Autodesk Inventor part; units mm, degrees
ref_plane "YZ Plane" through (0, 0, 0) normal (1, 0, 0) x (0, 1, 0)
ref_plane "XZ Plane" through (0, 0, 0) normal (0, 1, 0) x (-1, 0, 0)
ref_plane "XY Plane" through (0, 0, 0) normal (0, 0, 1) x (1, 0, 0)
sketch "Sketch1" plane through (0, 0, 0) normal (0, 0, 1) x (1, 0, 0)
  line L0 (-21.15, 15.4985) -> (-15.4985, 21.15)
  line L1 (-15.4985, 21.15) -> (15.4985, 21.15)
  line L2 (15.4985, 21.15) -> (21.15, 15.4985)
  line L3 (21.15, 15.4985) -> (21.15, -15.4985)
  line L4 (21.15, -15.4985) -> (15.4985, -21.15)
  line L5 (15.4985, -21.15) -> (-15.4985, -21.15)
  line L6 (-15.4985, -21.15) -> (-21.15, -15.4985)
  line L7 (-21.15, -15.4985) -> (-21.15, 15.4985)
  line L8 (28.575, -18.574) -> (28.575, 18.574)
  line L9 (28.575, 18.574) -> (18.574, 28.575)
  line L10 (18.574, 28.575) -> (-18.574, 28.575)
  line L11 (-18.574, 28.575) -> (-28.575, 18.574)
  line L12 (-28.575, 18.574) -> (-28.575, -18.574)
  line L13 (-28.575, -18.574) -> (-18.574, -28.575)
  line L14 (-18.574, -28.575) -> (18.574, -28.575)
  line L15 (18.574, -28.575) -> (28.575, -18.574)
  line L16 (-18.574, -28.575) -> (-145.574, -28.575)
  line L17 (-145.574, -28.575) -> (-145.574, 28.575)
  line L18 (-145.574, 28.575) -> (-18.574, 28.575)
  line L19 (-18.574, 28.575) -> (-18.574, -28.575)
  circle A0 centre (0, 0) radius 11
  point P0 (0, 0)
  dimension "d0" = 127
  dimension "d1" = 57.15
  dimension "d2" = 57.15
extrude "Extrusion1" add sketch "Sketch1" along normal blind 6.35 contours L7 L6 L19 L13 L12 L11 L0 | L0 L19 L6 L7 | L19 L10 L9 L8 L15 L14 L6 L5 L4 L3 L2 L1 L0 | L0 L1 L2 L3 L4 L5 L6 L19 | L11 L12 L13 L16 L17 L18 | A0
sketch "Sketch2" plane through (0, 0, 0) normal (0, 0, -1) x (-1, 0, 0)
  line L0 (130.4486, -16.3493) -> (130.4486, -9.9993)
  line L1 (126.7402, -9.9993) -> (126.7402, -16.3493)
  line L2 (130.4486, 9.0507) -> (130.4486, 15.4007)
  line L3 (126.7402, 15.4007) -> (126.7402, 9.0507)
  line L4 (126.7402, -12.7) -> (130.4486, -12.7) construction
  line L5 (126.7402, 12.7) -> (130.4486, 12.7) construction
  circle A0 centre (128.5944, -12.065) radius 1.8542
  circle A1 centre (128.5944, 12.065) radius 1.8542
  line L6 (-18.574, 28.575) -> (145.574, 28.575)
  line L7 (145.574, -28.575) -> (-18.574, -28.575)
  line L8 (242.583, -12.065) -> (-73.768, -12.065)
  dimension "d5" = 3.7084
  dimension "d6" = 3.7084
  dimension "d13" = 16.51
  dimension "d14" = 16.51
  dimension "d15" = 16.51
extrude "Extrusion2" cut sketch "Sketch2" against normal through all
sketch "Sketch3" plane through (0, 0, 0) normal (0, 0, -1) x (-1, 0, 0)
  line L0 (145.574, 28.575) -> (145.574, -28.575)
  line L1 (139.224, -24.0792) -> (145.574, -24.0792)
  line L2 (145.574, -28.575) -> (145.574, -24.0792)
  line L3 (-18.574, -28.575) -> (145.574, -28.575)
  line L4 (-28.575, -18.574) -> (-18.574, -28.575)
  line L5 (-28.575, 18.574) -> (-28.575, -18.574)
  line L6 (-18.574, 28.575) -> (-28.575, 18.574)
  line L7 (145.574, 28.575) -> (-18.574, 28.575)
  line L8 (145.574, 24.0792) -> (145.574, 28.575)
  line L9 (145.574, 24.0792) -> (139.224, 24.0792)
  line L10 (139.224, 24.0792) -> (139.224, 26.162)
  line L11 (139.224, 26.162) -> (136.43, 26.162)
  line L12 (136.43, 26.162) -> (136.43, 24.0792)
  line L13 (136.43, 24.0792) -> (132.874, 24.0792)
  line L14 (132.874, 24.0792) -> (132.874, 20.3708)
  line L15 (132.874, 20.3708) -> (136.43, 20.3708)
  line L16 (136.43, 20.3708) -> (136.43, 18.288)
  line L17 (136.43, 18.288) -> (139.224, 18.288)
  line L18 (139.224, 18.288) -> (139.224, 20.3708)
  line L19 (139.224, 20.3708) -> (145.574, 20.3708)
  line L20 (145.574, -20.3708) -> (145.574, 20.3708)
  line L21 (145.574, -20.3708) -> (139.224, -20.3708)
  line L22 (139.224, -20.3708) -> (139.224, -18.288)
  line L23 (139.224, -18.288) -> (136.43, -18.288)
  line L24 (136.43, -18.288) -> (136.43, -20.3708)
  line L25 (136.43, -20.3708) -> (132.874, -20.3708)
  line L26 (132.874, -20.3708) -> (132.874, -24.0792)
  line L27 (132.874, -24.0792) -> (136.43, -24.0792)
  line L28 (136.43, -24.0792) -> (136.43, -26.162)
  line L29 (136.43, -26.162) -> (139.224, -26.162)
  line L30 (139.224, -26.162) -> (139.224, -24.0792)
  circle A0 centre (128.5944, 12.7) radius 1.8542
  circle A1 centre (128.5944, -12.7) radius 1.8542
  circle A2 centre (-15.5, -15.5) radius 2
  circle A3 centre (15.5, -15.5) radius 2
  circle A4 centre (-15.5, 15.5) radius 2
  circle A5 centre (15.5, 15.5) radius 2
  circle A6 centre (0, 0) radius 11
extrude "Extrusion3" cut sketch "Sketch3" against normal through all contours L0 L19 L18 L17 L16 L15 L14 L13 L12 L11 L10 L9 | L0 L1 L30 L29 L28 L27 L26 L25 L24 L23 L22 L21
sketch "Sketch4" plane through (0, 0, 0) normal (0, 0, -1) x (-1, 0, 0)
  circle A0 centre (0, 0) radius 11
  circle A1 centre (0, 0) radius 19.05
  point P0 (0, 0)
  dimension "d24" = 38.1
  dimension "d25" = 22
extrude "Extrusion4" cut sketch "Sketch4" against normal through all contours A0 | A1
sketch "Sketch5" plane through (-145.574, -20.3708, 0) normal (-1, 0, 0) x (0, 0, 1)
  line L0 (0, 40.7416) -> (0, 0)
  line L1 (0, 33.0708) -> (0, 7.6708)
  line L2 (0, 7.6708) -> (6.35, 7.6708)
  line L3 (6.35, 7.6708) -> (6.35, 33.0708)
  line L4 (6.35, 33.0708) -> (0, 33.0708)
  point P0 (0, 20.3708)
extrude "Extrusion5" add sketch "Sketch5" along normal blind 6.35
sketch "Sketch6" plane through (0, 0, 6.35) normal (0, 0, 1) x (1, 0, 0)
  line L0 (-145.574, 28.575) -> (18.574, 28.575)
  circle A0 centre (-114.3, 38.1) radius 2.5146
  circle A1 centre (-114.3, -38.1) radius 2.5146
  line L1 (0, 50.8) -> (-127, 50.8)
  line L2 (-127, 50.8) -> (-127, -50.8)
  line L3 (-127, -50.8) -> (0, -50.8)
  line L4 (-127, 50.8) -> (-101.6, 50.8)
  line L5 (-101.6, 28.575) -> (-127, 28.575)
  line L6 (-127, 28.575) -> (-127, 50.8)
  spline S0 degree 4 poles (-101.6, 50.8) (-101.4278, 37.6809) (-93.5766, 28.9843) (-86.3032, 28.7086) (-77.2189, 28.575) knots 0 0 0 0 0 1 1 1 1 1
  line L7 (-101.6678, 55.9666) -> (-101.5322, 45.6334) construction
  arc A2 (-101.3699, 54.8975) -> (-101.2624, 46.71) centre (-71.935, 51.1893) ccw construction
  line L8 (-81.6682, 28.6405) -> (-72.7695, 28.5095) construction
  arc A3 (-80.7781, 28.6371) -> (-73.6593, 28.5323) centre (-67.6175, 681.2105) ccw construction
  line L9 (-151.924, 0) -> (28.575, 0) construction
  line L10 (0, -50.8) -> (-127, -50.8)
  line L11 (-101.6, -50.8) -> (-101.6, -28.575)
  line L12 (-127, -28.575) -> (-127, -50.8)
  spline S1 degree 4 poles (-101.6, -50.8) (-101.4278, -37.6809) (-93.5766, -28.9843) (-86.3032, -28.7086) (-77.2189, -28.575) knots 0 0 0 0 0 1 1 1 1 1
  line L13 (-101.6678, -55.9666) -> (-101.5322, -45.6334) construction
  arc A4 (-101.2624, -46.71) -> (-101.3699, -54.8975) centre (-71.935, -51.1893) ccw construction
  line L14 (-81.6682, -28.6405) -> (-72.7695, -28.5095) construction
  arc A5 (-73.6593, -28.5323) -> (-80.7781, -28.6371) centre (-67.6175, -681.2105) ccw construction
  line L15 (-77.2189, 28.575) -> (-101.6, 28.5129)
  point P0 (-91.9655, 31.5993)
  point P1 (-91.9655, -31.5993)
extrude "Extrusion6" add sketch "Sketch6" against normal blind 6.35 contours L2 L1 S0 L0
ref_plane "Work Plane1" through (-145.574, 0, 0) normal (0, -1, 0) x (1, 0, 0)
mirror "Mirror1" about plane through (-145.574, 0, 0) normal (0, -1, 0) of "Extrusion6"
sketch "Sketch7" plane through (0, 0, 0) normal (0, 0, -1) x (-1, 0, 0)
  line L0 (-28.575, 18.574) -> (-18.574, 28.575)
  line L1 (-18.574, -28.575) -> (-28.575, -18.574)
  line L2 (-28.575, -18.574) -> (-28.575, 18.574)
  line L3 (-60.325, -19.2943) -> (-48.1038, -19.2943)
  line L4 (-63.5, -16.1193) -> (-60.325, -19.2943)
  line L5 (-63.5, 16.1193) -> (-63.5, -16.1193)
  line L6 (-60.325, 19.2943) -> (-63.5, 16.1193)
  line L7 (-48.1038, 19.2943) -> (-60.325, 19.2943)
  line L8 (-48.1038, 19.2943) -> (-27.8548, 19.2943)
  line L9 (-48.1038, -19.2943) -> (-27.8548, -19.2943)
  circle A0 centre (-54.61, 0) radius 2.5146
extrude "Extrusion7" add sketch "Sketch7" against normal blind 6.35
sketch "Sketch8" plane through (0, 0, 0) normal (0, 0, -1) x (-1, 0, 0)
  circle A0 centre (50.8, 0) radius 3.175
extrude "Extrusion8" cut sketch "Sketch8" against normal through all
equation "\"d2\" = d1"
equation "\"d14\" = d13"
equation "\"d15\" = d14"
properties part number "tiltColumnStepperSide02_RB01" material "Gold"
The model under review builds one solid part; all positions refer to its coordinate system, in mm. A direction names the side the tool comes from. Coordinates: 2 decimals unless noted, no trailing zeros. Write each loop counter-clockwise with the first axis right and the second up, starting at its lowest first coordinate (ties: lowest second). Pieces come first, ordered by that corner, then holes. Notation, with made-up numbers: (-31.75, -28) - (2.25, -28) arc R28 cw to (2.25, 4) - close; hole circle Ø11 at (7.25, 16). An arc over 180 degrees is marked (long way). Answer in a Markdown table with one row per item. Add a question column.
Q1. To check wall thickness, follow line 1 along Y through (x, z) = (-133.5, 5.75) (3 decimals); line 2 along Y through (x, z) = (-50.5, 1) (3 decimals); line 3 along Y through (x, z) = (-114.3, 1.5). State the ranges of each line that lie inside material, in increasing order. Write a range as from..to.
Q2. Consider section C-C on x = -114.3. Give the boundary of the cut face in (y, z), then the cut area to 3 significant figures.
Q3. Clearance check with flat-ended pins moving along their axes: pin 1 (1.5 mm diameter, centred on x = -8, z = 3.5, fed in from -Y) (3 decimals); pin 2 (3 mm diameter, centred on x = -19, z = 2.5, fed in from +Y) (3 decimals); pin 3 (1.5 mm diameter, centred on x = -94.5, z = 1.5, fed in from -Y). State where each tip first meets the part, or that it passes through.
Q4. Consider section D-D on x = -72.5. Give the boundary of the cut face in (y, z) (3 decimals), then the cut area to 3 significant figures.
Q5. For faces 4 (the face through (-145.574, -26, 3)), 5 (the face through (-142, -20.371, 3)), 6 (the face through (44, 19.294, 3)), 7 (the face through (44, -19.294, 3)), list the 3-axis set-ups (+Z, -Z, +X, -X, +Y, -Y) from which the entire face can be reached by the end or side of a thin tool; tool diameter is ignored.
Q6. Draft analysis for pull direction Y (two halves, no side actions). For faces 1 (the face through (-30, -28.575, 3)), 2 (the face through (15.12, -11.59, 3.13)), 3 (the face through (-145.574, 16, 3)), state which applies: +Y half, -Y half, draft (parallel to the pull), parting line (faces both ways), or undercut.
Q7. Consider section B-B on y = 0. Give the boundary of the cut face in (x, z) (3 decimals).
Q8. Consider section A-A on x = -50.8. Give the boundary of the cut face in (y, z) (3 decimals), then the cut area to 3 significant figures.
Answers below:
| question | item | result |
|---|---|---|
| 1 | line 1 | -28.575..-24.079, -20.371..20.371, 24.079..28.575 |
| 1 | line 2 | -28.575..-3.161, 3.161..28.575 |
| 1 | line 3 | -50.8..-40.61, -35.59..35.59, 40.61..50.8 |
| 2 | outline | (-50.8, 0) - (-40.61, 0) - (-40.61, 6.35) - (-50.8, 6.35) - close; (-35.59, 0) - (35.59, 0) - (35.59, 6.35) - (-35.59, 6.35) - close; (40.61, 0) - (50.8, 0) - (50.8, 6.35) - (40.61, 6.35) - close |
| 2 | area | 581 mm² |
| 3 | pin 1 | y = -28.575 |
| 3 | pin 2 | y = 28.575 |
| 3 | pin 3 | y = -34.19 |
| 4 | outline | (-28.575, 0) - (28.575, 0) - (28.575, 6.35) - (-28.575, 6.35) - close |
| 4 | area | 363 mm² |
| 5 | face 4 | +Z, -Z, -X, -Y |
| 5 | face 5 | +Z, -Z, -X |
| 5 | face 6 | +Z, -Z, +X, +Y |
| 5 | face 7 | +Z, -Z, +X, -Y |
| 6 | face 1 | -Y half |
| 6 | face 2 | undercut |
| 6 | face 3 | draft |
| 7 | outline | (-151.924, 0) - (-53.975, 0) - (-53.975, 6.35) - (-151.924, 6.35) - close; (-47.625, 0) - (-19.05, 0) - (-19.05, 6.35) - (-47.625, 6.35) - close; (19.05, 0) - (52.095, 0) - (52.095, 6.35) - (19.05, 6.35) - close; (57.125, 0) - (63.5, 0) - (63.5, 6.35) - (57.125, 6.35) - close |
| 8 | outline | (-28.575, 0) - (-3.175, 0) - (-3.175, 6.35) - (-28.575, 6.35) - close; (3.175, 0) - (28.575, 0) - (28.575, 6.35) - (3.175, 6.35) - close |
| 8 | area | 323 mm² |
